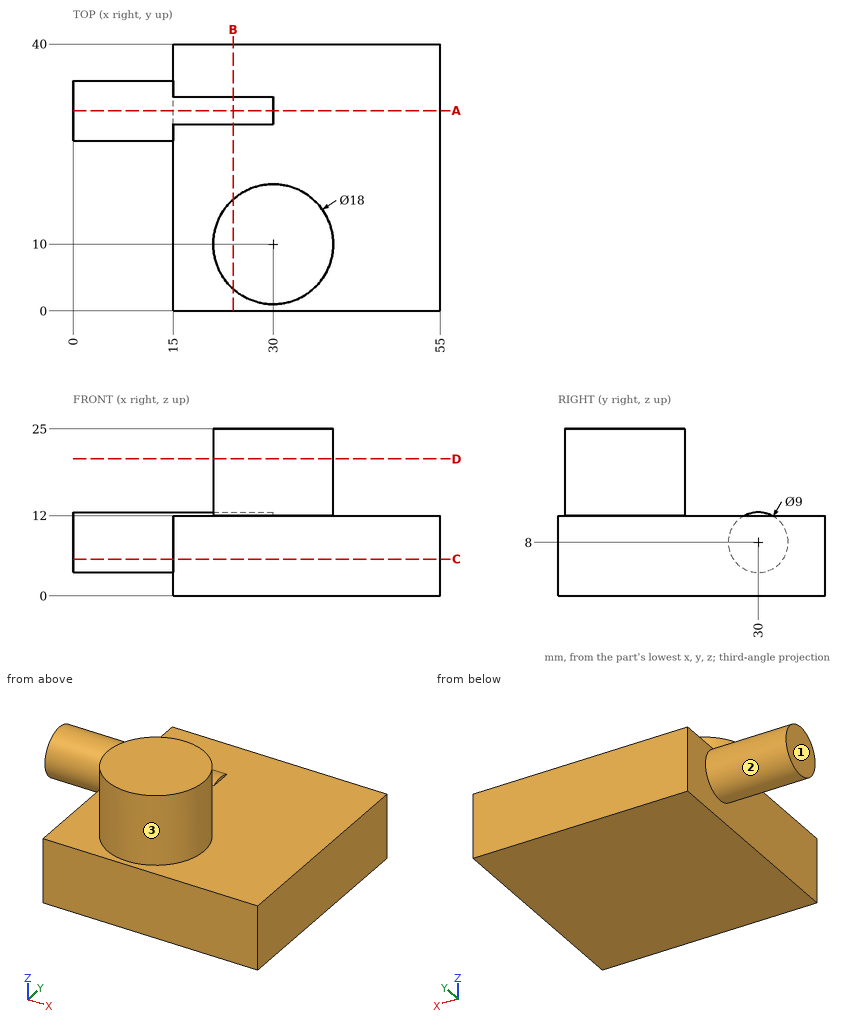
The figure shows three views and two pictorial views of one solid part (mm, origin at its lowest corner). Answer the questions. A direction names the side the tool comes from. Coordinates: 2 decimals unless noted, no trailing zeros. Write each loop counter-clockwise with the first axis right and the second up, starting at its lowest first coordinate (ties: lowest second). Pieces come first, ordered by that corner, then holes.
1. The part is cut by section B-B, the plane x = 24. Write down the section's boundary in (y, z), and give its area (3 significant figures).
Results list:
outline: (0, 0) - (40, 0) - (40, 12) - (32.06, 12) arc R4.5 ccw to (27.94, 12) - (16.71, 12) - (16.71, 25) - (3.29, 25) - (3.29, 12) - (0, 12) - close
area: 656 mm2
2. Consider line 1 along X through (y, z) = (9.5, 12.75); line 2 along Z through (x, y) = (42, 14); line 3 along X through (y, z) = (19, 2.75). Determine where each line is inside the solid, lowest interval first.
Results list:
line 1: x = 21.01 to 38.99
line 2: z = 0 to 12
line 3: x = 15 to 55
3. For the marked faces 1, 2 and 3, determine the directions among +Z, -Z, +X, -X, +Y, -Y from which every point of the face is accessible in a straight line to the end or side of a thin tool.
Results list:
face 1: +Z, -Z, -X, +Y, -Y
face 2: -X
face 3: +Z
4. Flat-ended cylindrical pins translate along their axes: pin 1 (3 mm diameter, centred on x = 24, y = 19, fed in from +Z); pin 2 (10 mm diameter, centred on y = 13.5, z = 14.5, fed in from -X); pin 3 (10 mm diameter, centred on x = 24.5, z = 18, fed in from +Y). Find the tip coordinate at first contact, or state that the pin passes through.
Results list:
pin 1: stops at z = 12
pin 2: stops at x = 15
pin 3: stops at y = 18.99
5. The part is cut by section D-D, the plane z = 20.5. Write down the section's boundary in (x, y).
Results list:
outline: circle Ø18 at (30, 10)
6. The part is cut by section A-A, the plane y = 30. Write down the section's boundary in (x, z).
Results list:
outline: (0, 3.5) - (15, 3.5) - (15, 0) - (55, 0) - (55, 12) - (30, 12) - (30, 12.5) - (0, 12.5) - close
7. The part is cut by section C-C, the plane z = 5.5. Write down the section's boundary in (x, y), and give its area (3 significant figures).
Results list:
outline: (0, 26.26) - (15, 26.26) - (15, 0) - (55, 0) - (55, 40) - (15, 40) - (15, 33.74) - (0, 33.74) - close
area: 1,710 mm2
